Verification items for the finished model (mm, model axes). A direction names the side the tool comes from. Give positions to 0.01 mm unless a question says otherwise; leave off trailing zeros. Loops run counter-clockwise (first coordinate to the right, second up) from the corner with the lowest first, then second, coordinate; pieces in that order, holes last. Notation, with made-up numbers: M 74,79.5 L 118,79.5 A20 ccw 118,103.5 Z; hole C 24,58 d2. An arc over 180 degrees is marked long. Put each result on its own line as item: value. Start each with the question number.
from build123d import *

# Parameters (mm, degrees)
ESQUISSE1_R             = 21
BOSS_EXTRU_1_DEPTH      = 50
ESQUISSE2_R             = 32.5
BOSS_EXTRU_2_DEPTH      = 5
ESQUISSE3_R             = 18.5
ENL_V_MAT_EXTRU_1_DEPTH = 12
ESQUISSE4_R             = 6
ENL_V_MAT_EXTRU_2_DEPTH = 49
ENL_V_START             = -12
ESQUISSE5_R             = 18.5
ENL_V_MAT_EXTRU_3_DEPTH = 12
ESQUISSE6_R             = 2
ENL_V_MAT_EXTRU_4_DEPTH = 6


with BuildPart() as part:
    # Esquisse1 → Boss.-Extru.1 (new body)
    with BuildSketch(Plane.XY):
        Circle(ESQUISSE1_R)
    extrude(amount=BOSS_EXTRU_1_DEPTH)

    # Esquisse2 → Boss.-Extru.2 (add)
    with BuildSketch(Plane.XY.offset(50)):
        Circle(ESQUISSE2_R)
    extrude(amount=BOSS_EXTRU_2_DEPTH)

    # Esquisse3 → Enlèv. mat.-Extru.1 (cut)
    with BuildSketch(Plane.XY.offset(55)):
        Circle(ESQUISSE3_R)
    extrude(amount=-ENL_V_MAT_EXTRU_1_DEPTH, mode=Mode.SUBTRACT)

    # Esquisse4 → Enlèv. mat.-Extru.2 (cut)
    with BuildSketch(Plane.XY.offset(43)):
        Circle(ESQUISSE4_R)
    extrude(amount=-ENL_V_MAT_EXTRU_2_DEPTH, mode=Mode.SUBTRACT)

    # Esquisse5 → Enlèv. mat.-Extru.3 (cut)
    with BuildSketch(Plane(origin=(0, 0, 0), x_dir=(-1, 0, 0), z_dir=(0, 0, -1)).offset(ENL_V_START)):
        with Locations(Location((0, 0, 0), (0, 0, 180))):
            Circle(ESQUISSE5_R)
    extrude(amount=ENL_V_MAT_EXTRU_3_DEPTH, mode=Mode.SUBTRACT)

    # Esquisse6 → Enlèv. mat.-Extru.4 (cut)
    with BuildSketch(Plane(origin=(0, 0, 50), x_dir=(-1, 0, 0), z_dir=(0, 0, -1))):
        with Locations((27, 0)):
            Circle(ESQUISSE6_R)
        with Locations((-27, 0)):
            Circle(ESQUISSE6_R)
    extrude(amount=-ENL_V_MAT_EXTRU_4_DEPTH, mode=Mode.SUBTRACT)


solid = part.part
Q1. Release check for a two-part mould opening along Y. For faces 4 (the face through (31, 9.76, 52.46)), 5 (the face through (-4.01, -18.06, 49.08)), 6 (the face through (14, -14, 55)) record: pulls with the +Y half, pulls with the -Y half, needs draft (parallel to the pull), parting line crosses it, or undercut.
Q2. Cross-section at A-A, the plane x = 0. Record the boundary of the cut face in (y, z), then the cut area to 4 significant figures.
Q3. Set-up check for faces 1 (the face through (-0.5, -21.2, 50)), 2 (the face through (-6, 0, 28)), 3 (the face through (-4.4, 4.4, 43)): record each of +Z, -Z, +X, -X, +Y, -Y from which the full face is reachable in a straight line by a thin tool's end or side.
Q4. Go/stop test with flat-tipped pins: pin 1 (3 mm diameter, centred on x = 9, z = 7.5, fed in from -Y); pin 2 (2 mm diameter, centred on x = -8.5, y = -23.5, fed in from -Z); pin 3 (1 mm diameter, centred on y = 1.5, z = 43.5, fed in from -X). Record where each tip stops, or that it passes through.
Q5. Cross-section at B-B, the plane y = 0. Record the boundary of the cut face in (x, z).
Q6. Cross-section at C-C, the plane z = 4. Record the boundary of the cut face in (x, y), then the cut area to 3 significant figures.
Q7. Cross-section at D-D, the plane y = -12.5. Record the boundary of the cut face in (x, z), then the cut area to 3 significant figures.
Q8. Scan lines: L1, parallel to Y at x = 0, z = 51; L2, parallel to X at y = -0.5, z = 21; L3, parallel to Y at x = 0, z = 46. Record each from-to range of solid material in increasing order.
Ans:
1. face 4: parting line crosses it
1. face 5: undercut
1. face 6: needs draft
2. outline: M -32.5,50 L -21,50 L -21,0 L -18.5,0 L -18.5,12 L -6,12 L -6,43 L -18.5,43 L -18.5,55 L -32.5,55 Z; M 6,12 L 18.5,12 L 18.5,0 L 21,0 L 21,50 L 32.5,50 L 32.5,55 L 18.5,55 L 18.5,43 L 6,43 Z
2. area: 1,165 mm^2
3. face 1: -Z
3. face 2: +Z, -Z
3. face 3: +Z
4. pin 1: stops at y = -19.62
4. pin 2: stops at z = 50
4. pin 3: stops at x = -20.98
5. outline: M -32.5,50 L -29,50 L -29,55 L -32.5,55 Z; M -25,50 L -21,50 L -21,0 L -18.5,0 L -18.5,12 L -6,12 L -6,43 L -18.5,43 L -18.5,55 L -25,55 Z; M 6,12 L 18.5,12 L 18.5,0 L 21,0 L 21,50 L 25,50 L 25,55 L 18.5,55 L 18.5,43 L 6,43 Z; M 29,50 L 32.5,50 L 32.5,55 L 29,55 Z
6. outline: C 0,0 d42; hole C 0,0 d37
6. area: 310 mm^2
7. outline: M -30,50 L -16.87,50 L -16.87,0 L -13.64,0 L -13.64,12 L 13.64,12 L 13.64,0 L 16.87,0 L 16.87,50 L 30,50 L 30,55 L 13.64,55 L 13.64,43 L -13.64,43 L -13.64,55 L -30,55 Z
7. area: 1,330 mm^2
8. L1: y = -32.5 to -18.5, 18.5 to 32.5
8. L2: x = -20.99 to -5.98, 5.98 to 20.99
8. L3: y = -21 to -18.5, 18.5 to 21
